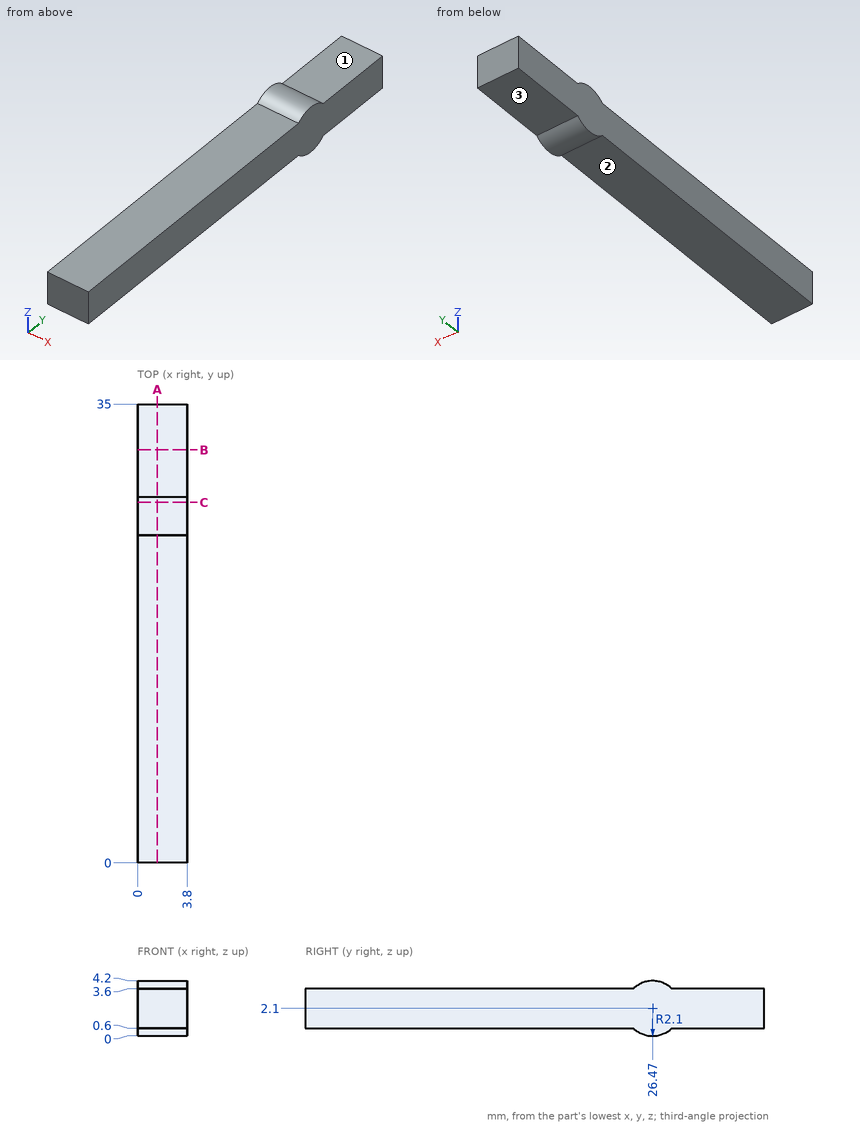
Part print with two shaded views. Sizes in mm from the minimum x, y, z corner. A direction names the side the tool comes from. Coordinates: 2 decimals unless noted, no trailing zeros. Write each loop counter-clockwise with the first axis right and the second up, starting at its lowest first coordinate (ties: lowest second). Pieces come first, ordered by that corner, then holes. Notation, with made-up numbers: M 27.25,89 L 43.25,89 A14 ccw 43.25,93 Z; hole C 83,39.5 d2. An arc over 180 degrees is marked long. Return JSON: item names as keys, results as strings.
Item 1: Slice it at B-B, the plane y = 31.5. Write the cut outline in (x, z), and give its area (3 significant figures).
Findings below:
{"outline": "M 0,0.6 L 3.8,0.6 L 3.8,3.6 L 0,3.6 Z", "area": "11.4 mm2"}
Item 2: Slice it at A-A, the plane x = 1.5. Write the cut outline in (y, z).
Findings below:
{"outline": "M 0,0.6 L 25,0.6 A2.1 ccw 27.94,0.6 L 35,0.6 L 35,3.6 L 27.94,3.6 A2.1 ccw 25,3.6 L 0,3.6 Z"}
Item 3: Drop flat-ended pins along their axis: pin 1 Ø1.5 at (x, y) = (2, 19.5) entering from -Z; pin 2 Ø1.1 at (x, y) = (1.5, 31.5) entering from +Z. Give the stop position or say it passes through.
Findings below:
{"pin 1": "stops at z = 0.6", "pin 2": "stops at z = 3.6"}
Item 4: Slice it at C-C, the plane y = 27.5. Write the cut outline in (x, z).
Findings below:
{"outline": "M 0,0.27 L 3.8,0.27 L 3.8,3.93 L 0,3.93 Z"}
Item 5: Probe line 1 (Z direction, x = 1.05, y = 32); line 2 (Y direction, x = 0.35, z = 3.65) (1 decimal); line 3 (Y direction, x = 2.35, z = 3.7). List the from-to ranges inside material, lowest first. Write a range as from..to.
Findings below:
{"line 1": "z = 0.6..3.6", "line 2": "y = 25.1..27.9", "line 3": "y = 25.11..27.83"}
Item 6: Which spindle directions (+Z, -Z, +X, -X, +Y, -Y) get a long thin tool onto all of the face, cutting with end or side? Do the marked faces 1, 2 and 3. Say none if no direction does.
Findings below:
{"face 1": "+Z, +X, -X, +Y", "face 2": "-Z, +X, -X, -Y", "face 3": "-Z, +X, -X, +Y"}
